```python
from build123d import *

# Parameters (mm, degrees)
SKETCH1_R           = 11.25
SKETCH1_R_2         = 1.5
BOSS_EXTRUDE1_DEPTH = 11.3
SKETCH4_W           = 34.3
SKETCH4_H           = 11.3
BOSS_EXTRUDE3_DEPTH = 5
BOSS_EXTRUDE4_DEPTH = 11.3
SKETCH6_W           = 34.3
SKETCH6_H           = 133
BOSS_EXTRUDE5_DEPTH = 11.3
BOSS_EXTRUDE6_DEPTH = 133
CUT_EXTRUDE1_DEPTH  = 121.7
BOSS_EXTRUDE8_DEPTH = 2.65
BOSS_EXTRUDE9_DEPTH = 2.65
SKETCH13_R          = 4.7625
CUT_EXTRUDE2_DEPTH  = 137.719320142
SKETCH14_W          = 23.3
SKETCH14_H          = 8.15
CUT_EXTRUDE3_DEPTH  = 9.43
CUT_EXTRUDE4_DEPTH  = 2.65


with BuildPart() as part:
    # Sketch1 → Boss-Extrude1 (new body)
    with BuildSketch(Plane(origin=(0, 0, 0), x_dir=(1, 0, 0), z_dir=(0, 1, 0))):
        Polygon((-21.15, 17.15), (-17.15, 21.15), (17.15, 21.15), (21.15, 17.15), (21.15, -17.15), (17.15, -21.15), (-17.15, -21.15), (-21.15, -17.15), align=None)
        with Locations(Location((0, 0, 0), (0, 0, 270))):
            Circle(SKETCH1_R, mode=Mode.SUBTRACT)
        with Locations(Location((-15.5, 15.5, 0), (0, 0, 270))):
            Circle(SKETCH1_R_2, mode=Mode.SUBTRACT)
        with Locations(Location((15.5, 15.5, 0), (0, 0, 270))):
            Circle(SKETCH1_R_2, mode=Mode.SUBTRACT)
        with Locations(Location((15.5, -15.5, 0), (0, 0, 270))):
            Circle(SKETCH1_R_2, mode=Mode.SUBTRACT)
        with Locations(Location((-15.5, -15.5, 0), (0, 0, 270))):
            Circle(SKETCH1_R_2, mode=Mode.SUBTRACT)
    extrude(amount=BOSS_EXTRUDE1_DEPTH)

    # Sketch4 → Boss-Extrude3 (add)
    with BuildSketch(Plane(origin=(0, 0, -21.15), x_dir=(-1, 0, 0), z_dir=(0, 0, -1))):
        with Locations((0, 5.65)):
            Rectangle(SKETCH4_W, SKETCH4_H)
    extrude(amount=BOSS_EXTRUDE3_DEPTH)

    # Sketch5 → Boss-Extrude4 (add)
    with BuildSketch(Plane(origin=(0, 11.3, 0), x_dir=(1, 0, 0), z_dir=(0, 1, 0))):
        Polygon((21.15, 17.15), (17.15, 26.15), (17.15, 21.15), align=None)
        Polygon((-17.15, 26.15), (-21.15, 17.15), (-17.15, 21.15), align=None)
    extrude(amount=-BOSS_EXTRUDE4_DEPTH)

    # Sketch6 → Boss-Extrude5 (add)
    with BuildSketch(Plane(origin=(0, 0, -26.15), x_dir=(-1, 0, 0), z_dir=(0, 0, -1))):
        with Locations((0, -55.2)):
            Rectangle(SKETCH6_W, SKETCH6_H)
    extrude(amount=BOSS_EXTRUDE5_DEPTH)

    # Sketch9 → Boss-Extrude6 (add)
    with BuildSketch(Plane(origin=(0, 11.3, 0), x_dir=(1, 0, 0), z_dir=(0, 1, 0))):
        Polygon((21.15, 17.15), (21.15, 37.45), (17.15, 37.45), (17.15, 26.15), align=None)
        Polygon((-17.15, 37.45), (-17.15, 26.15), (-21.15, 17.15), (-21.15, 37.45), align=None)
    extrude(amount=-BOSS_EXTRUDE6_DEPTH)

    # Sketch10 → Cut-Extrude1 (cut)
    with BuildSketch(Plane.XZ.offset(121.7)):
        Polygon((-17.15, -26.15), (-21.15, -17.15), (-21.15, -26.15), align=None)
        Polygon((17.15, -26.15), (21.15, -17.15), (21.15, -26.15), align=None)
    extrude(amount=-CUT_EXTRUDE1_DEPTH, mode=Mode.SUBTRACT)

    # Sketch11 → Boss-Extrude8 (add)
    with BuildSketch(Plane.ZY.offset(18.5)):
        Polygon((-26.15, -38.3), (12.15, 0), (-12.15, 0), (-26.15, -14), align=None)
    extrude(amount=BOSS_EXTRUDE8_DEPTH)

    # Sketch12 → Boss-Extrude9 (add)
    with BuildSketch(Plane(origin=(21.15, 0, 0), x_dir=(0, 0, -1), z_dir=(1, 0, 0))):
        Polygon((-12.15, 0), (12.15, 0), (26.15, -14), (26.15, -38.3), align=None)
    extrude(amount=-BOSS_EXTRUDE9_DEPTH)

    # Sketch13 → Cut-Extrude2 (cut, through all)
    with BuildSketch(Plane(origin=(0, 0, -37.45), x_dir=(-1, 0, 0), z_dir=(0, 0, -1))):
        with Locations((8, -69.2)):
            Circle(SKETCH13_R)
        with Locations((-8, -69.2)):
            Circle(SKETCH13_R)
        with Locations((8, -99.2)):
            Circle(SKETCH13_R)
        with Locations((-8, -99.2)):
            Circle(SKETCH13_R)
    extrude(amount=-CUT_EXTRUDE2_DEPTH, mode=Mode.SUBTRACT)

    # Sketch14 → Cut-Extrude3 (cut)
    with BuildSketch(Plane.XZ):
        with Locations((0, 17.075)):
            Rectangle(SKETCH14_W, SKETCH14_H)
    extrude(amount=-CUT_EXTRUDE3_DEPTH, mode=Mode.SUBTRACT)

    # Sketch15 → Cut-Extrude4 (cut)
    with BuildSketch(Plane.ZY.offset(21.15)):
        Polygon((-22.8566684, -35.0066684), (-22.8566684, -24.211458174), (-12.061458174, -24.211458174), align=None)
    extrude(amount=-CUT_EXTRUDE4_DEPTH, mode=Mode.SUBTRACT)


solid = part.part
```
For this review, take the finished solid that the model builds, in its own axes (mm). A direction names the side the tool comes from. Round coordinates to 2 decimals unless told otherwise and drop trailing zeros. Loops run counter-clockwise (first coordinate to the right, second up) from the corner with the lowest first, then second, coordinate; pieces in that order, holes last.
(1) Clearance check with flat-ended pins moving along their axes: P1, Ø2, axis at x = 14, z = 7.5, coming from the -Y side; P2, Ø4.5, axis at x = 2.5, y = 7, coming from the +Z side; P3, Ø2.5, axis at x = -5.5, z = 19, coming from the -Y side. State where each tip first meets the part, or that it passes through.
Returned:
P1: stops at y = 0
P2: stops at z = 13
P3: stops at y = 9.43
(2) We need section D-D (x = 0). Give the boundary of the cut face in (y, z), plus the area to 3 significant figures.
Returned:
outline: (-121.7, -37.45) - (11.3, -37.45) - (11.3, -11.25) - (0, -11.25) - (0, -26.15) - (-121.7, -26.15) - close; (0, 11.25) - (11.3, 11.25) - (11.3, 21.15) - (9.43, 21.15) - (9.43, 13) - (0, 13) - close
area: 1,710 mm2
(3) Mouldability with a two-part tool opening along Z and no side actions: class faces 4 (the flat face through (-19.81, -6.9, -19.05)), 5 (the flat face through (4, 11, 21.15)), 6 (the cylindrical face through (-15.43, 5.57, -17)), 7 (the cylindrical face through (-12.4, -71.02, -31.88)) as released by +Z, released by -Z, zero draft, split by the parting line, or undercut.
Returned:
face 4: undercut
face 5: released by +Z
face 6: undercut
face 7: zero draft
(4) We need section C-C (y = -99.2). Give the boundary of the cut face in (x, z), plus the area to 3 significant figures.
Returned:
outline: (-21.15, -37.45) - (-12.76, -37.45) - (-12.76, -26.15) - (-21.15, -26.15) - close; (-3.24, -37.45) - (3.24, -37.45) - (3.24, -26.15) - (-3.24, -26.15) - close; (12.76, -37.45) - (21.15, -37.45) - (21.15, -26.15) - (12.76, -26.15) - close
area: 263 mm2
(5) Tool access review of faces 1 (the cylindrical face through (-4.31, 5.57, 10.39)), 2 (the flat face through (18.5, -15, -12)), 3 (the flat face through (-20, -30, -22.857)): name each direction out of +Z, -Z, +X, -X, +Y, -Y from which nothing blocks a thin tool from reaching the whole face with its end or side.
Returned:
face 1: +Y, -Y
face 2: +Z, -Y
face 3: +Z, -X, -Y
(6) Wall thickness on line 1 along Y through (x, z) = (8, -34); line 2 along Z through (x, y) = (-15, 4); line 3 along X through (y, z) = (3, 15): over which ranges is each line inside the solid? List them lowest first.
Returned:
line 1: y = -121.7 to -103.96, -94.44 to -73.96, -64.44 to 11.3
line 2: z = -37.45 to -16.91, -14.09 to 14.09, 16.91 to 21.15
line 3: x = -21.15 to -16.91, -14.09 to -11.65, 11.65 to 14.09, 16.91 to 21.15
(7) We need section B-B (x = 15.5). Give the boundary of the cut face in (y, z), plus the area to 3 significant figures.
Returned:
outline: (-121.7, -37.45) - (11.3, -37.45) - (11.3, -17) - (0, -17) - (0, -26.15) - (-121.7, -26.15) - close; (0, -14) - (11.3, -14) - (11.3, 14) - (0, 14) - close; (0, 17) - (11.3, 17) - (11.3, 21.15) - (0, 21.15) - close
area: 1,970 mm2
(8) We need section A-A (z = -19). Give the boundary of the cut face in (x, y), plus the area to 3 significant figures.
Returned:
outline: (-21.15, -24.21) - (-18.5, -24.21) - (-18.5, -6.85) - (-21.15, -6.85) - close; (-21.15, 0) - (21.15, 0) - (21.15, 11.3) - (-21.15, 11.3) - close; (18.5, -31.15) - (21.15, -31.15) - (21.15, -6.85) - (18.5, -6.85) - close
area: 588 mm2
